```python
from build123d import *

# Parameters (mm, degrees)
SKETCH1_R           = 2.5
BOSS_EXTRUDE1_DEPTH = 10
BOSS_EXTRUDE2_DEPTH = 2
BOSS_EXTRUDE3_DEPTH = 2
CHAMFER1_SIZE       = 0.7


with BuildPart() as part:
    # Sketch1 → Boss-Extrude1 (new body)
    with BuildSketch(Plane(origin=(0, 0, 0), x_dir=(1, 0, 0), z_dir=(0, 1, 0))):
        Circle(SKETCH1_R)
    extrude(amount=BOSS_EXTRUDE1_DEPTH)

    # Sketch3 → Boss-Extrude2 (add)
    with BuildSketch(Plane.XZ):
        Polygon((3.421887709, 0), (1.710943854, 2.963441685), (-1.710943854, 2.963441685), (-3.421887709, 0), (-1.710943854, -2.963441685), (1.710943854, -2.963441685), align=None)
    extrude(amount=BOSS_EXTRUDE2_DEPTH)

    # Sketch2 → Boss-Extrude3 (add)
    with BuildSketch(Plane(origin=(0, 10, 0), x_dir=(1, 0, 0), z_dir=(0, 1, 0))):
        Polygon((3.421887709, 0), (1.710943854, 2.963441685), (-1.710943854, 2.963441685), (-3.421887709, 0), (-1.710943854, -2.963441685), (1.710943854, -2.963441685), align=None)
    extrude(amount=BOSS_EXTRUDE3_DEPTH)

    # Chamfer1
    chamfer1_edges = [part.edges().sort_by_distance(p)[0] for p in [
        (0, 12, -2.963441685),
        (-2.566415782, 12, -1.481720842),
        (-2.566415782, 12, 1.481720842),
        (0, 12, 2.963441685),
        (2.566415782, 12, 1.481720842),
        (2.566415782, 12, -1.481720842),
        (2.566415782, -2, -1.481720842),
        (2.566415782, -2, 1.481720842),
        (0, -2, 2.963441685),
        (-2.566415782, -2, 1.481720842),
        (-2.566415782, -2, -1.481720842),
        (0, -2, -2.963441685),
    ]]
    chamfer(chamfer1_edges, length=CHAMFER1_SIZE)


solid = part.part
```
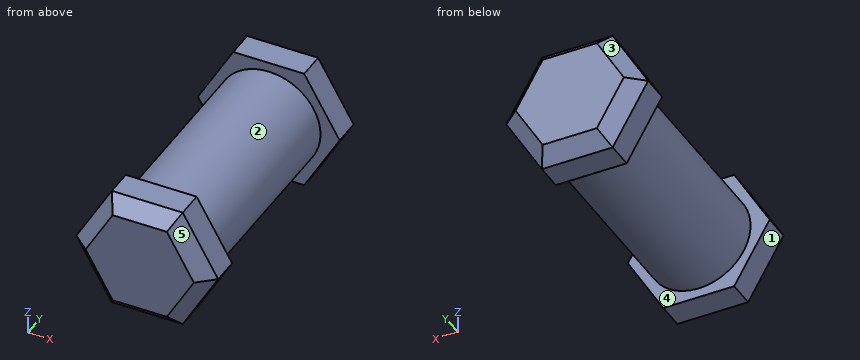
Design review of the part built by this model. Coordinates are the model's own, in mm. Face numbers are marked on the shaded views. A direction names the side the tool comes from. Coordinates: 2 decimals unless noted, no trailing zeros. Write each loop counter-clockwise with the first axis right and the second up, starting at its lowest first coordinate (ties: lowest second). Pieces come first, ordered by that corner, then holes.
1) Machinability: for the marked faces 4 and 5, which of the approach directions +Z, -Z, +X, -X, +Y, -Y give a long, thin tool a straight path to every point of the face, cutting with its end or side? Answer none if there is none.
2) Mouldability with a two-part tool opening along Y and no side actions: class the marked faces 1, 2 and 3 as +Y half, -Y half, draft (parallel to the pull), parting line (faces both ways), or undercut.
3) Add section A-A (x = 0). Write out the cut boundary in (y, z).
4) Add section B-B (y = 2.5). Write out the cut boundary in (x, z).
5) Add section C-C (z = 1.6). Write out the cut boundary in (x, y), plus the area to 3 significant figures.
6) To check wall thickness, follow L1, parallel to Y at x = -1.25, z = 2.2; L2, parallel to Y at x = 2.25, z = 1.7; L3, parallel to X at y = 3.75, z = -0.05. State the ranges of each line that lie inside material, in increasing order.
Check result:
1. face 4: none
1. face 5: +Z, +X, -Y
2. face 1: draft
2. face 2: undercut
2. face 3: +Y half
3. outline: (-2, -2.26) - (-1.3, -2.96) - (0, -2.96) - (0, -2.5) - (10, -2.5) - (10, -2.96) - (11.3, -2.96) - (12, -2.26) - (12, 2.26) - (11.3, 2.96) - (10, 2.96) - (10, 2.5) - (0, 2.5) - (0, 2.96) - (-1.3, 2.96) - (-2, 2.26) - close
4. outline: circle Ø5 at (0, 0)
5. outline: (-2.5, -1.3) - (-1.69, -2) - (1.69, -2) - (2.5, -1.3) - (2.5, 0) - (1.92, 0) - (1.92, 10) - (2.5, 10) - (2.5, 11.3) - (1.69, 12) - (-1.69, 12) - (-2.5, 11.3) - (-2.5, 10) - (-1.92, 10) - (-1.92, 0) - (-2.5, 0) - close
5. area: 57.3 mm2
6. L1: y = -2 to 0, 10 to 12
6. L2: y = -1.46 to 0, 10 to 11.46
6. L3: x = -2.5 to 2.5
